from build123d import *

# Parameters (mm, degrees)
F1_DEPTH = 5.84
F2_W     = 2.79
F2_H     = 0.66
F3_DEPTH = 1.875


with BuildPart() as f1:
    # F0 (on Front) → F1 (new body)
    with BuildSketch(Plane.XZ):
        with BuildLine():
            ThreePointArc((1.5338823529, 3.8022631323), (0, -4.1), (-1.5338823529, 3.8022631323))
            ThreePointArc((-1.5338823529, 3.8022631323), (-1.4656664827, 3.8574586018), (-1.44, 3.9413703201))
            Line((-1.44, 3.9413703201), (-1.44, 4.2738156254))
            ThreePointArc((-1.44, 4.2738156254), (-1.5044003351, 4.3969931289), (-1.6423026316, 4.4144016657))
            ThreePointArc((-1.6423026316, 4.4144016657), (0, -4.71), (1.6423026316, 4.4144016657))
            ThreePointArc((1.6423026316, 4.4144016657), (1.5044003351, 4.3969931289), (1.44, 4.2738156254))
            Line((1.44, 4.2738156254), (1.44, 3.9413703201))
            ThreePointArc((1.44, 3.9413703201), (1.4656664827, 3.8574586018), (1.5338823529, 3.8022631323))
        make_face()
    extrude(amount=F1_DEPTH)

    # F2 (on Right) → F3 (join, symmetric)
    with BuildSketch(Plane.YZ):
        with Locations((1.395, -4.41)):
            Rectangle(F2_W, F2_H)
        with BuildLine():
            Line((2.79, -4.08), (2.79, -4.74))
            ThreePointArc((2.79, -4.74), (3.5399175523, -5.4788795349), (2.8122384852, -6.2396702274))
            ThreePointArc((2.8122384852, -6.2396702274), (2.79, -6.24), (2.7677615148, -6.2396702274))
            Line((2.7677615148, -6.2396702274), (-28.9377615148, -6.2396702274))
            ThreePointArc((-28.9377615148, -6.2396702274), (-29.2889547374, -5.9627547168), (-29.1015934199, -5.5566579103))
            ThreePointArc((-29.1015934199, -5.5566579103), (-25.9439060993, -4.8439864519), (-22.8290893137, -5.7253525592))
            ThreePointArc((-22.8290893137, -5.7253525592), (-22.363124468, -5.613733552), (-22.4985094857, -5.154110949))
            ThreePointArc((-22.4985094857, -5.154110949), (-25.9261622728, -4.1842250127), (-29.4009912886, -4.9684734867))
            ThreePointArc((-29.4009912886, -4.9684734867), (-29.9307497668, -6.1166999675), (-28.9377615148, -6.8996702274))
            Line((-28.9377615148, -6.8996702274), (2.7595065561, -6.8996702274))
            ThreePointArc((2.7595065561, -6.8996702274), (4.1999175544, -5.5052476135), (2.79, -4.08))
        make_face()
        with BuildLine():
            ThreePointArc((2.7677615148, -6.2396702274), (2.79, -6.24), (2.8122384852, -6.2396702274))
            Line((2.8122384852, -6.2396702274), (2.7677615148, -6.2396702274))
        make_face()
    extrude(amount=F3_DEPTH, both=True)


solid = f1.part
Geometry check sheet. Reference: the model listing, model coordinates, mm. A direction names the side the tool comes from. Coordinates: 2 decimals unless noted, no trailing zeros. Order: outer loops, then holes, each group sorted by start corner. A loop starts at its lowest first (then second) coordinate and runs counter-clockwise, first axis right, second up. Notation, with made-up numbers: M 0.5,-33.5 L 43.5,-33.5 A21 ccw 43.5,-14.5 Z; hole C 16,48 d6. An arc over 180 degrees is marked long. Use CSV: the item, a comma, the result in double quotes.
Item 1: Cross-section at D-D on y = -11.5. Record the cut outline in (x, z) (3 decimals), then the cut area to 4 significant figures.
Returned:
outline,"M -1.875,-6.9 L 1.875,-6.9 L 1.875,-6.24 L -1.875,-6.24 Z"
area,"2.475 mm2"
Item 2: Tool access check on faces 1 (the flat face through (0, 1, -4.08)), 2 (the cylindrical face through (0.026, -25.876, -4.186)), 3 (the flat face through (0, -13, -6.24)). Record the directions out of +Z, -Z, +X, -X, +Y, -Y that give a thin tool (end or side, any length) a straight path to the whole face; none if there is none.
Returned:
face 1,"+Z, +X, -X, +Y"
face 2,"+Z, +X, -X"
face 3,"+X, -X"
Item 3: Cross-section at A-A on z = 0. Record the cut outline in (x, y), then the cut area to 3 significant figures.
Returned:
outline,"M -4.71,-5.84 L -4.1,-5.84 L -4.1,0 L -4.71,0 Z; M 4.1,-5.84 L 4.71,-5.84 L 4.71,0 L 4.1,0 Z"
area,"7.12 mm2"
Item 4: Thickness scan on line 1 along Z through (x, y) = (0, -2.5); line 2 along X through (y, z) = (-2.6, 0); line 3 along Y through (x, z) = (-1.75, -4). Record the ranges inside material, lowest first.
Returned:
line 1,"z = -6.9 to -6.24, -4.71 to -4.1"
line 2,"x = -4.71 to -4.1, 4.1 to 4.71"
line 3,"y = -5.84 to 0"
Item 5: Mould release check, pull along Z, two halves, no side actions. Record for faces 4 (the flat face through (0, -13, -6.9)), 5 (the cylindrical face through (0.026, -29.935, -6.098)), 6 (the cylindrical face through (0.026, -25.99, -4.843)): pulls with the +Z half, pulls with the -Z half, needs draft (parallel to the pull), parting line crosses it, or undercut.
Returned:
face 4,"pulls with the -Z half"
face 5,"parting line crosses it"
face 6,"undercut"
Item 6: Cross-section at B-B on x = 2.5. Record the cut outline in (y, z).
Returned:
outline,"M -5.84,-3.99 L 0,-3.99 L 0,-3.25 L -5.84,-3.25 Z; M -5.84,3.25 L 0,3.25 L 0,3.99 L -5.84,3.99 Z"
Item 7: Gauge pin test, flat ends, axial feed: pin 1 Ø1.5 at (x, y) = (3.5, -25.5) entering from +Z; pin 2 Ø5 at (x, y) = (3, -23) entering from +Z; pin 3 Ø4.5 at (x, z) = (3.5, 0) entering from +Y; pin 4 Ø1 at (x, y) = (3, -1) entering from -Z. Record the tip position at first contact, or that the pin passes through.
Returned:
pin 1,"passes through"
pin 2,"stops at z = -4.24"
pin 3,"stops at y = 0"
pin 4,"stops at z = -3.99"
